from build123d import *

# Parameters (mm, degrees)
SKETCH1_W           = 110
SKETCH1_H           = 150
BOSS_EXTRUDE1_DEPTH = 10
CUT_EXTRUDE1_DEPTH  = 6
SKETCH3_R           = 2.5
BOSS_EXTRUDE2_DEPTH = 18
CUT_EXTRUDE2_START  = -12
SKETCH5_R           = 1.1
CUT_EXTRUDE2_DEPTH  = 5
CUT_EXTRUDE3_START  = 0.5
CUT_EXTRUDE3_DEPTH  = 4
SKETCH7_R           = 1.875
BOSS_EXTRUDE3_DEPTH = 11.5
CUT_EXTRUDE4_DEPTH  = 4
SKETCH9_W           = 10
SKETCH9_H           = 11.4
BOSS_EXTRUDE4_DEPTH = 10
SKETCH10_R          = 3
CUT_EXTRUDE5_DEPTH  = 161.819432905
SKETCH11_W          = 4.5
SKETCH11_H          = 18
BOSS_EXTRUDE5_DEPTH = 3
FILLET1_R           = 2


with BuildPart() as part:
    # Sketch1 → Boss-Extrude1 (new body)
    with BuildSketch(Plane.XY):
        with Locations((55, 75)):
            Rectangle(SKETCH1_W, SKETCH1_H)
    extrude(amount=BOSS_EXTRUDE1_DEPTH)

    # Sketch2 → Cut-Extrude1 (cut)
    with BuildSketch(Plane(origin=(0, 0, 0), x_dir=(-1, 0, 0), z_dir=(0, 0, -1))):
        with BuildLine():
            Line((-93, 53), (-7, 53))
            ThreePointArc((-7, 53), (-5.585786438, 53.585786438), (-5, 55))
            Line((-5, 55), (-5, 113))
            ThreePointArc((-5, 113), (-5.585786438, 114.414213562), (-7, 115))
            Line((-7, 115), (-93, 115))
            ThreePointArc((-93, 115), (-94.414213562, 114.414213562), (-95, 113))
            Line((-95, 113), (-95, 55))
            ThreePointArc((-95, 55), (-94.414213562, 53.585786438), (-93, 53))
        make_face()
    extrude(amount=-CUT_EXTRUDE1_DEPTH, mode=Mode.SUBTRACT)

    # Sketch3 → Boss-Extrude2 (add)
    with BuildSketch(Plane(origin=(0, 0, 6), x_dir=(-1, 0, 0), z_dir=(0, 0, -1))):
        with Locations(Location((-91.46, 95.2, 0), (0, 0, 180))):
            Circle(SKETCH3_R)
        with Locations(Location((-70.96, 111.2, 0), (0, 0, 180))):
            Circle(SKETCH3_R)
        with Locations(Location((-9.46, 110.2, 0), (0, 0, 180))):
            Circle(SKETCH3_R)
        with Locations(Location((-9.46, 76.2, 0), (0, 0, 180))):
            Circle(SKETCH3_R)
        with Locations(Location((-24.96, 58.2, 0), (0, 0, 180))):
            Circle(SKETCH3_R)
        with Locations(Location((-51.96, 58.2, 0), (0, 0, 180))):
            Circle(SKETCH3_R)
        with Locations(Location((-91.46, 58.2, 0), (0, 0, 180))):
            Circle(SKETCH3_R)
    extrude(amount=BOSS_EXTRUDE2_DEPTH)

    # Sketch5 → Cut-Extrude2 (cut)
    with BuildSketch(Plane.XY.offset(CUT_EXTRUDE2_START)):
        with Locations(Location((91.46, 58.2, 0), (0, 0, 180))):
            Circle(SKETCH5_R)
        with Locations(Location((51.96, 58.2, 0), (0, 0, 180))):
            Circle(SKETCH5_R)
        with Locations(Location((24.96, 58.2, 0), (0, 0, 180))):
            Circle(SKETCH5_R)
        with Locations(Location((9.46, 76.2, 0), (0, 0, 180))):
            Circle(SKETCH5_R)
        with Locations(Location((9.46, 110.2, 0), (0, 0, 180))):
            Circle(SKETCH5_R)
        with Locations(Location((70.96, 111.2, 0), (0, 0, 180))):
            Circle(SKETCH5_R)
        with Locations(Location((91.46, 95.2, 0), (0, 0, 180))):
            Circle(SKETCH5_R)
    extrude(amount=CUT_EXTRUDE2_DEPTH, mode=Mode.SUBTRACT)

    # Sketch6 → Cut-Extrude3 (cut)
    with BuildSketch(Plane(origin=(0, 0, 6), x_dir=(-1, 0, 0), z_dir=(0, 0, -1)).offset(CUT_EXTRUDE3_START)):
        with BuildLine():
            Line((-87.5, 78), (-83.5, 78))
            ThreePointArc((-83.5, 78), (-82.085786438, 78.585786438), (-81.5, 80))
            Line((-81.5, 80), (-81.5, 91))
            ThreePointArc((-81.5, 91), (-82.085786438, 92.414213562), (-83.5, 93))
            Line((-83.5, 93), (-87.5, 93))
            ThreePointArc((-87.5, 93), (-88.914213562, 92.414213562), (-89.5, 91))
            Line((-89.5, 91), (-89.5, 80))
            ThreePointArc((-89.5, 80), (-88.914213562, 78.585786438), (-87.5, 78))
        make_face()
    extrude(amount=-CUT_EXTRUDE3_DEPTH, mode=Mode.SUBTRACT)

    # Sketch7 → Boss-Extrude3 (add)
    with BuildSketch(Plane(origin=(0, 0, 6), x_dir=(-1, 0, 0), z_dir=(0, 0, -1))):
        with Locations(Location((-32.95, 88.15, 0), (0, 0, 180))):
            Circle(SKETCH7_R)
    extrude(amount=BOSS_EXTRUDE3_DEPTH)

    # Sketch8 → Cut-Extrude4 (cut)
    with BuildSketch(Plane.XY.offset(10)):
        with BuildLine():
            Line((30.7, 78.15), (30.7, 85.469048676))
            ThreePointArc((30.7, 85.469048676), (32.95, 91.65), (35.2, 85.469048676))
            Line((35.2, 85.469048676), (35.2, 78.15))
            Line((35.2, 78.15), (35.5, 78.15))
            Line((35.5, 78.15), (35.5, 85.332643083))
            ThreePointArc((35.5, 85.332643083), (32.95, 91.95), (30.4, 85.332643083))
            Line((30.4, 85.332643083), (30.4, 78.15))
            Line((30.4, 78.15), (30.7, 78.15))
        make_face()
    extrude(amount=-CUT_EXTRUDE4_DEPTH, mode=Mode.SUBTRACT)

    # Sketch9 → Boss-Extrude4 (add)
    with BuildSketch(Plane.ZY):
        with Locations((5, 39)):
            Rectangle(SKETCH9_W, SKETCH9_H)
        with Locations((5, 111)):
            Rectangle(SKETCH9_W, SKETCH9_H)
    extrude(amount=BOSS_EXTRUDE4_DEPTH)

    # Sketch10 → Cut-Extrude5 (cut, through all)
    with BuildSketch(Plane(origin=(0, 116.7, 0), x_dir=(1, 0, 0), z_dir=(0, 1, 0))):
        with Locations(Location((-5, -5, 0), (0, 0, 270))):
            Circle(SKETCH10_R)
    extrude(amount=-CUT_EXTRUDE5_DEPTH, mode=Mode.SUBTRACT)

    # Sketch11 → Boss-Extrude5 (add)
    with BuildSketch(Plane(origin=(110, 0, 0), x_dir=(0, 0, -1), z_dir=(1, 0, 0))):
        with Locations((-5, 75)):
            Rectangle(SKETCH11_W, SKETCH11_H)
    extrude(amount=BOSS_EXTRUDE5_DEPTH)

    # Fillet1
    fillet1_edges = [part.edges().sort_by_distance(p)[0] for p in [
        (0, 150, 5),
        (110, 150, 5),
        (110, 0, 5),
        (0, 0, 5),
    ]]
    fillet(fillet1_edges, radius=FILLET1_R)


solid = part.part
Build history of the part. All positions in model axes, mm. A direction names the side the tool comes from. Round coordinates to 2 decimals unless told otherwise and drop trailing zeros. Write each loop counter-clockwise with the first axis right and the second up, starting at its lowest first coordinate (ties: lowest second). Pieces come first, ordered by that corner, then holes. Notation, with made-up numbers: M 89,57 L 131,57 A9 cw 131,66 Z; hole C -11,6.5 d3. An arc over 180 degrees is marked long. Answer as a JSON object with one key per item and string values. Group by question number.
(1) Flat gauge pins, fed straight in: pin 1 (1.5 mm diameter, centred on x = 112, z = 5.5, fed in from -Y); pin 2 (2 mm diameter, centred on x = 56.5, z = -6, fed in from -Y); pin 3 (2 mm diameter, centred on x = 58, y = 88.5, fed in from -Z); pin 4 (3 mm diameter, centred on x = -3, z = 3.5, fed in from +Y). Where does each tip first touch, or does it go through?
(2) Which spindle directions (+Z, -Z, +X, -X, +Y, -Y) get a long thin tool onto all of the face, cutting with end or side? Do faces 4 (the flat face through (111, 84, 5)), 5 (the flat face through (111, 75, 2.75)), 6 (the cylindrical face through (73.345, 110.449, -2.874)). Say none if no direction does.
(3) Mould opens along X. For faces 1 (the flat face through (-2.7, 116.7, 2.7)), 2 (the flat face through (0, 17, 5)), 3 (the cylindrical face through (9.13, 73.72, -2.87)) say: pulls with the +X half, pulls with the -X half, needs draft (parallel to the pull), parting line crosses it, or undercut.
(4) Cut at A-A (y = 88.15). Give the cut face in (x, z) (3 decimals).
(5) Drill centre lines: L1, parallel to X at y = 88.15, z = 8.55; L2, parallel to X at y = 58.2, z = -10.8; L3, parallel to Y at x = 51.96, z = -10.9. Where is each one in solid material? Low to high.
(6) Cut at D-D (y = 70.5). Give the cut face in (x, z).
(7) Cut at C-C (x = 14.5). Give the cut face in (y, z).
(8) Cut at B-B (x = -5). Give the cut face in (y, z).
Responses:
{
 "1": {"pin 1": "stops at y = 66", "pin 2": "passes through", "pin 3": "stops at z = 6", "pin 4": "stops at y = 116.7"},
 "2": {"face 4": "+Z, -Z, +X, +Y", "face 5": "-Z, +X, +Y, -Y", "face 6": "-Z"},
 "3": {"face 1": "needs draft", "face 2": "pulls with the -X half", "face 3": "undercut"},
 "4": {"outline": "M 0,0 L 5,0 L 5,6 L 29.15,6 L 29.15,10 L 0,10 Z; M 29.45,6 L 31.075,6 L 31.075,-5.5 L 34.825,-5.5 L 34.825,6 L 36.45,6 L 36.45,10 L 29.45,10 Z; M 36.75,6 L 81.5,6 L 81.5,9.5 L 89.5,9.5 L 89.5,6 L 95,6 L 95,0 L 110,0 L 110,10 L 36.75,10 Z"},
 "5": {"L1": "x = 0 to 29.15, 29.45 to 36.45, 36.75 to 81.5, 89.5 to 110", "L2": "x = 22.46 to 23.86, 26.06 to 27.46, 49.46 to 50.86, 53.06 to 54.46, 88.96 to 90.36, 92.56 to 93.96", "L3": "y = 55.7 to 57.1, 59.3 to 60.7"},
 "6": {"outline": "M 0,0 L 5,0 L 5,6 L 95,6 L 95,0 L 110,0 L 110,2.75 L 113,2.75 L 113,7.25 L 110,7.25 L 110,10 L 0,10 Z"},
 "7": {"outline": "M 0,0 L 53,0 L 53,6 L 115,6 L 115,0 L 150,0 L 150,10 L 0,10 Z"},
 "8": {"outline": "M 33.3,0 L 44.7,0 L 44.7,2 L 33.3,2 Z; M 33.3,8 L 44.7,8 L 44.7,10 L 33.3,10 Z; M 105.3,0 L 116.7,0 L 116.7,2 L 105.3,2 Z; M 105.3,8 L 116.7,8 L 116.7,10 L 105.3,10 Z"}
}
